Build history of the part. All positions in model axes, mm. Face numbers are marked on the shaded views. Give positions to 0.01 mm unless a question says otherwise; leave off trailing zeros. Loops run counter-clockwise (first coordinate to the right, second up) from the corner with the lowest first, then second, coordinate; pieces in that order, holes last. Notation, with made-up numbers: M -22,71.25 L -8,71.25 A23 ccw -8,103.25 Z; hole C -38,45.5 d10. An arc over 180 degrees is marked long. Answer as a JSON object with one key per item and string values. Group by question number.
1. Slice it at A-A (y = 30). List the corners of the cut face in (x, z).
2. Drill centre lines: line 1 along Y through (x, z) = (30, -7.75); line 2 along Y through (x, z) = (20, -7.5). Where is each one in solid material? Low to high. Write a range as [from, to].
3. Drop a flat-ended pin along its axis: pin 1 Ø12 at (x, y) = (48.5, 34) entering from +Z. Give the stop position or say it passes through.
4. Slice it at C-C (z = -14). List the corners of the cut face in (x, y), then the cut area to 3 significant figures.
5. Mould opens along Y. For the marked faces 1, 2 and 3 say: released by +Y, released by -Y, zero draft, split by the parting line, or undercut.
from build123d import *

# Parameters (mm, degrees)
SKETCH_1_W      = 60
SKETCH_1_H      = 60
SKETCH_1_R      = 11
EXTRUDE_1_DEPTH = 20
CHAMFER_1_SIZE  = 2


with BuildPart() as part:
    # Эскиз1 → Бобышка-Вытянуть1 (new body)
    with BuildSketch(Plane.XY):
        with Locations((30, 30)):
            Rectangle(SKETCH_1_W, SKETCH_1_H)
        with Locations((30, 30)):
            Circle(SKETCH_1_R, mode=Mode.SUBTRACT)
    extrude(amount=-EXTRUDE_1_DEPTH)

    # Фаска1
    chamfer_1_edges = [part.edges().sort_by_distance(p)[0] for p in [
        (19, 30, -20),
        (19, 30, 0),
    ]]
    chamfer(chamfer_1_edges, length=CHAMFER_1_SIZE)


solid = part.part
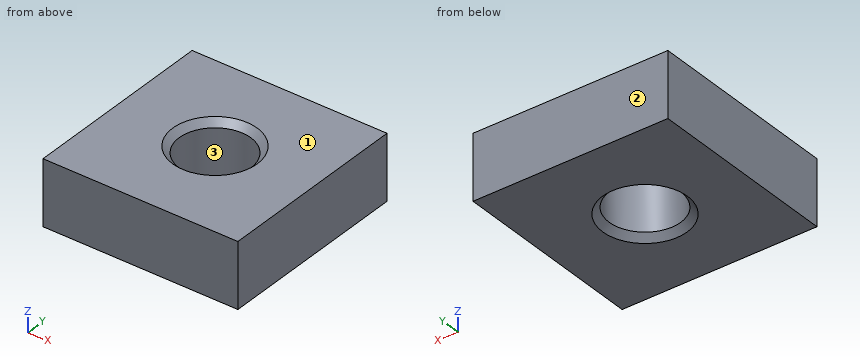
Established:
{
 "1": {"outline": "M 0,-20 L 17,-20 L 19,-18 L 19,-2 L 17,0 L 0,0 Z; M 41,-18 L 43,-20 L 60,-20 L 60,0 L 43,0 L 41,-2 Z"},
 "2": {"line 1": "y = [0, 19], [41, 60]", "line 2": "y = [0, 25.42], [34.58, 60]"},
 "3": {"pin 1": "stops at z = 0"},
 "4": {"outline": "M 0,0 L 60,0 L 60,60 L 0,60 Z; hole C 30,30 d22", "area": "3,220 mm^2"},
 "5": {"face 1": "zero draft", "face 2": "released by +Y", "face 3": "undercut"}
}
